```python
from build123d import *

# Parameters (mm, degrees)
F0_W     = 304.8
F0_H     = 152.4
F1_DEPTH = 12.7
F2_R     = 11.622867
F2_R_2   = 12.321487
F2_R_3   = 12.818207
F2_R_4   = 12.730774
F3_DEPTH = 12.7


with BuildPart() as f1:
    # F0 (on Top) → F1 (new body, symmetric)
    with BuildSketch(Plane.XY):
        Rectangle(F0_W, F0_H)
    extrude(amount=F1_DEPTH, both=True)

    # F2 (on Top) → F3 (cut, symmetric)
    with BuildSketch(Plane.XY):
        with Locations((-133.876547, 56.070849)):
            Circle(F2_R)
        with Locations((-132.619306, -58.75669)):
            Circle(F2_R_2)
        with Locations((125.533119, 56.070849)):
            Circle(F2_R_3)
        with Locations((125.952214, -54.984987)):
            Circle(F2_R_4)
    extrude(amount=F3_DEPTH, both=True, mode=Mode.SUBTRACT)


solid = f1.part
```
Geometry: final body of the model. Coordinates: model frame, mm. Round coordinates to 2 decimals unless told otherwise and drop trailing zeros. Order: outer loops, then holes, each group sorted by start corner. A loop starts at its lowest first (then second) coordinate and runs counter-clockwise, first axis right, second up. Notation, with made-up numbers: (66.25, -4.5) -> (111.25, -4.5) arc R28 cw to (111.25, 26.5) -> close; hole circle Ø9 at (43, 82.25). An arc over 180 degrees is marked (long way). Use CSV: the item, a comma, the result in double quotes. Start each with the question number.
1) Material intervals for line 1 along X through (y, z) = (57, 5.5); line 2 along Y through (x, z) = (-140, 3.25); line 3 along X through (y, z) = (64, 3.25), sorted ascending. Write a range as from..to.
2) Section B-B (z = -8.5). Return the cut outline in (x, y), and give its area (3 significant figures).
3) Section A-A (y = 51). Return the cut outline in (x, z), and give its area (3 significant figures).
4) Draft query along X for faces 1 (the face through (152.4, -1, 0)), 2 (the face through (137.712, -59.861, 0.178)), 3 (the face through (-2, 1, 12.7)). Return one class per face: +X half, -X half, draft (parallel to the pull), parting line (faces both ways), or undercut.
5) First-contact query: pin 1 Ø15.5 at (x, y) = (125.53, 56.07) entering from -Z. Flat tip, straight axial feed; report the tip coordinate or a pass-through.
Returned:
1,line 1,"x = -152.4..-145.46, -122.29..112.75, 138.32..152.4"
1,line 2,"y = -76.2..-68.62, -48.89..46.19, 65.95..76.2"
1,line 3,"x = -152.4..-142.37, -125.38..115.46, 135.6..152.4"
2,outline,"(-152.4, -76.2) -> (152.4, -76.2) -> (152.4, 76.2) -> (-152.4, 76.2) -> close; hole circle Ø23.25 at (-133.88, 56.07); hole circle Ø24.64 at (-132.62, -58.76); hole circle Ø25.64 at (125.53, 56.07); hole circle Ø25.46 at (125.95, -54.98)"
2,area,"44,500 mm²"
3,outline,"(-152.4, -12.7) -> (-144.33, -12.7) -> (-144.33, 12.7) -> (-152.4, 12.7) -> close; (-123.42, -12.7) -> (113.76, -12.7) -> (113.76, 12.7) -> (-123.42, 12.7) -> close; (137.31, -12.7) -> (152.4, -12.7) -> (152.4, 12.7) -> (137.31, 12.7) -> close"
3,area,"6,610 mm²"
4,face 1,"+X half"
4,face 2,"undercut"
4,face 3,"draft"
5,pin 1,"passes through"
